Read the model definition and answer for the solid it produces. Units are mm, in the model's axes. Face numbers are marked on the shaded views. A direction names the side the tool comes from. Coordinates: 2 decimals unless noted, no trailing zeros. Loops run counter-clockwise (first coordinate to the right, second up) from the corner with the lowest first, then second, coordinate; pieces in that order, holes last. Notation, with made-up numbers: (70, 15.25) - (82, 15.25) arc R20 cw to (82, 33.25) - close; hole circle Ø10 at (-22, 44). An arc over 180 degrees is marked (long way). Use one line per item in the form item = value.
from build123d import *

# Parameters (mm, degrees)
EXTRUDE_1_DEPTH = 13


with BuildPart() as part:
    # Эскиз1 → Бобышка-Вытянуть1 (new body)
    with BuildSketch(Plane.XY):
        Polygon((-4.461885495, 0), (3.788114505, 0), (7.163114505, 3), (7.163114505, 4.5), (3.663114505, 4.5), (3.663114505, 5.5), (-4.336885495, 5.5), (-4.336885495, 4.5), (-7.836885495, 4.5), (-7.836885495, 3), align=None)
    extrude(amount=EXTRUDE_1_DEPTH)

    # Эскиз4 → Зенковка для  винта с плоской головкой M52 (revolve, cut)
    with BuildSketch(Plane(origin=(-0.471799648, 5.5, 6.859193471), x_dir=(0, 0, 1), z_dir=(1, 0, 0))):
        Polygon((0, 0), (0, 5.5), (2.75, 5.5), (2.75, 2.45), (2.75, 0), align=None)
    revolve(axis=Axis((-0.471799648, 11.85, 6.859193471), (0, -1, 0)), mode=Mode.SUBTRACT)


solid = part.part
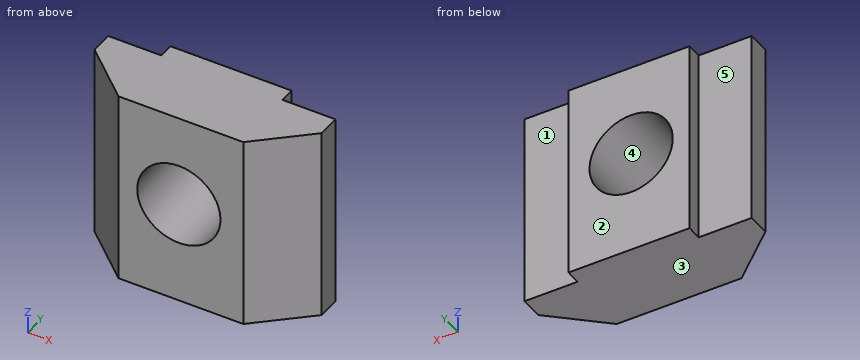
Item 1: The part is cut by section C-C on y = 2.1. Give the vertices of the cut face in (x, z), plus the area to 3 significant figures.
Results below:
outline = (-6.82, 0) - (6.15, 0) - (6.15, 13) - (-6.82, 13) - close; hole circle Ø5.5 at (-0.47, 6.86)
area = 145 mm²
Item 2: Which of the six approach directions +Z, -Z, +X, -X, +Y, -Y give full straight-line access (tool end or side, diameter ignored) to the marked faces 1 and 2?
Results below:
face_1 = +Z, -Z, +X, +Y
face_2 = +Z, -Z, +X, -X, +Y
Item 3: The part is cut by section B-B on x = 1.75. Give the vertices of the cut face in (y, z), plus the area to 3 significant figures.
Results below:
outline = (0, 0) - (5.5, 0) - (5.5, 5.24) - (0, 5.24) - close; (0, 8.48) - (5.5, 8.48) - (5.5, 13) - (0, 13) - close
area = 53.7 mm²
Item 4: Each of these flat-tipped pins is pushed along its axis until it touches: P1, Ø1.8, axis at x = -6, z = 9.5, coming from the +Y side; P2, Ø0.8, axis at y = 5, z = 6, coming from the +X side; P3, Ø0.5, axis at y = 5, z = 8.5, coming from the -X side. Where does it stop, or does it pass through?
Results below:
P1 = 4.5
P2 = 3.66
P3 = -4.34
Item 5: For a pull along Z with two mould halves and no side action, classify the marked faces 3, 4 and 5 as +Z half, -Z half, draft (parallel to the pull), parting line (faces both ways), or undercut.
Results below:
face_3 = -Z half
face_4 = undercut
face_5 = draft
Item 6: The part is cut by section A-A on z = 5.75. Give the vertices of the cut face in (x, y).
Results below:
outline = (-7.84, 3) - (-4.46, 0) - (-2.99, 0) - (-2.99, 5.5) - (-4.34, 5.5) - (-4.34, 4.5) - (-7.84, 4.5) - close; (2.04, 0) - (3.79, 0) - (7.16, 3) - (7.16, 4.5) - (3.66, 4.5) - (3.66, 5.5) - (2.04, 5.5) - close
Item 7: Find the intervals of material crossed by L1, parallel to X at y = 2.8, z = 5; L2, parallel to X at y = 4.7, z = 8.75; L3, parallel to Z at x = 1.5, y = 1.3, in increasing order.
Results below:
L1 = -7.61 to -2.5, 1.55 to 6.94
L2 = -4.34 to -2.47, 1.53 to 3.66
L3 = 0 to 4.94, 8.78 to 13
Item 8: The part is cut by section D-D on z = 10.75. Give the vertices of the cut face in (x, y).
Results below:
outline = (-7.84, 3) - (-4.46, 0) - (3.79, 0) - (7.16, 3) - (7.16, 4.5) - (3.66, 4.5) - (3.66, 5.5) - (-4.34, 5.5) - (-4.34, 4.5) - (-7.84, 4.5) - close
